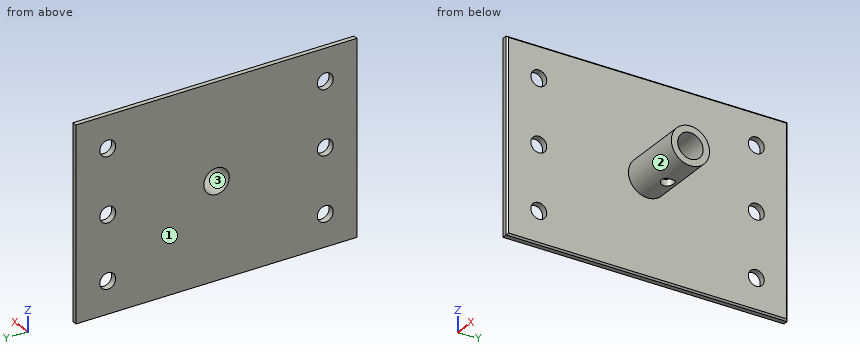
Autodesk Inventor part; units mm, degrees
ref_plane "Work Plane1" through (2, 0, -6) normal (0, 0, -1) x (-1, 0, 0)
ref_plane "YZ Plane" through (0, 0, 0) normal (1, 0, 0) x (0, 1, 0)
ref_plane "XZ Plane" through (0, 0, 0) normal (0, 1, 0) x (-1, 0, 0)
sketch "Sketch1" plane through (0, 0, 0) normal (1, 0, 0) x (0, 1, 0)
  line L0 (44.15, 30) -> (-44.15, 30)
  line L1 (-44.15, 30) -> (-44.15, -30)
  line L2 (-44.15, -30) -> (44.15, -30)
  line L3 (44.15, -30) -> (44.15, 30)
  line L4 (44.15, 30) -> (-44.15, -30) construction
  line L5 (-44.15, 30) -> (44.15, -30) construction
  circle A0 centre (0, 0) radius 4
  circle A1 centre (0, 0) radius 6
  line L6 (44.15, 30) -> (44.15, 20)
  line L7 (44.15, 20) -> (34.15, 20)
  line L8 (44.15, -30) -> (44.15, -20)
  line L9 (44.15, -20) -> (34.15, -20)
  line L10 (-44.15, 30) -> (-44.15, 20)
  line L11 (-44.15, 20) -> (-34.15, 20)
  line L12 (-44.15, -30) -> (-44.15, -20)
  line L13 (-44.15, -20) -> (-34.15, -20)
  line L14 (-44.15, 0) -> (-34.15, 0)
  line L15 (44.15, 0) -> (34.15, 0)
  circle A2 centre (34.15, 20) radius 2.5
  circle A3 centre (34.15, 0) radius 2.5
  circle A4 centre (34.15, -20) radius 2.5
  circle A5 centre (-34.15, 20) radius 2.5
  circle A6 centre (-34.15, 0) radius 2.5
  circle A7 centre (-34.15, -20) radius 2.5
  dimension "d0" = 88.3
  dimension "d1" = 60
  dimension "d2" = 8
  dimension "d3" = 12
  dimension "d4" = 10
  dimension "d5" = 10
  dimension "d6" = 10
  dimension "d7" = 10
  dimension "d8" = 10
  dimension "d9" = 10
  dimension "d10" = 10
  dimension "d11" = 10
  dimension "d12" = 10
  dimension "d13" = 10
  dimension "d14" = 5
  dimension "d15" = 5
  dimension "d16" = 5
  dimension "d17" = 5
  dimension "d18" = 5
  dimension "d19" = 5
extrude "Extrusion1" add sketch "Sketch1" along normal blind 2 contours L3 L2 L1 L0
sketch "Sketch2" plane through (2, 0, 0) normal (1, 0, 0) x (0, 0, -1)
  circle A0 centre (0, 0) radius 6
  circle A1 centre (0, 0) radius 4
  dimension "d22" = 12
  dimension "d23" = 8
extrude "Extrusion2" add sketch "Sketch2" along normal blind 21 and the other way blind 2
ref_plane "Work Plane1" through (2, 0, -6) normal (0, 0, -1) x (-1, 0, 0)
sketch "Sketch3" plane through (2, 0, -6) normal (0, 0, -1) x (-1, 0, 0)
  line L0 (-21, 6) -> (-21, -6)
  line L1 (-21, 0) -> (-10, 0)
  circle A0 centre (-10, 0) radius 2
  point P0 (2, 0)
  dimension "d28" = 11
  dimension "d29" = 4
extrude "Extrusion3" cut sketch "Sketch3" against normal blind 5
thread "Thread1"
chamfer "Chamfer1" distance 0.5 angle 45 4 edges at (2, 44.15, 0) (2, 0, -30) (2, 0, 30) (2, -44.15, 0)
properties part number "ax4_holder" material "Iron, Malleable"
Here's how the part is built. I have some questions about the finished solid (model axes, mm). Face numbers are marked on the shaded views. Coordinates: 2 decimals unless noted, no trailing zeros. Loops run counter-clockwise (first coordinate to the right, second up) from the corner with the lowest first, then second, coordinate; pieces in that order, holes last. Notation, with made-up numbers: M -23.5,75 L -0.5,75 A16 cw -0.5,104 Z; hole C 52.5,54.5 d10. An arc over 180 degrees is marked long. One line per item, written item: value.
1. Imagine slicing it at D-D (y = -9). List the corners of the cut face in (x, z) for me, and give its area (3 significant figures).
Geometry says:
outline: M 0,-30 L 1.5,-30 L 2,-29.5 L 2,29.5 L 1.5,30 L 0,30 Z
area: 120 mm2
2. Thinking about a two-plate mould opening in Y: for the marked faces 1, 2 and 3, which applies, +Y half, -Y half, draft (parallel to the pull), parting line (faces both ways), or undercut?
Geometry says:
face 1: draft
face 2: parting line
face 3: undercut
3. Will these pins go through, and if not, where does the flat tip stop? pin 1 Ø4 at (y, z) = (21, 17.5) entering from +X; pin 2 Ø1.5 at (x, z) = (3, 5) entering from -Y; pin 3 Ø4.5 at (x, y) = (12, 0) entering from -Z; pin 4 Ø6.5 at (y, z) = (34.15, 20) entering from -X.
Geometry says:
pin 1: stops at x = 2
pin 2: stops at y = -4.24
pin 3: stops at z = -6
pin 4: stops at x = 0
4. Imagine slicing it at C-C (z = 20). List the corners of the cut face in (x, y) for me, and give its area (3 significant figures).
Geometry says:
outline: M 0,-44.15 L 1.5,-44.15 L 2,-43.65 L 2,-36.65 L 0,-36.65 Z; M 0,-31.65 L 2,-31.65 L 2,31.65 L 0,31.65 Z; M 0,36.65 L 2,36.65 L 2,43.65 L 1.5,44.15 L 0,44.15 Z
area: 156 mm2
5. Imagine slicing it at A-A (y = -34.15). List the corners of the cut face in (x, z) for me.
Geometry says:
outline: M 0,-30 L 1.5,-30 L 2,-29.5 L 2,-22.5 L 0,-22.5 Z; M 0,-17.5 L 2,-17.5 L 2,-2.5 L 0,-2.5 Z; M 0,2.5 L 2,2.5 L 2,17.5 L 0,17.5 Z; M 0,22.5 L 2,22.5 L 2,29.5 L 1.5,30 L 0,30 Z
6. Imagine slicing it at B-B (z = 0). List the corners of the cut face in (x, y) for me.
Geometry says:
outline: M 0,-44.15 L 1.5,-44.15 L 2,-43.65 L 2,-36.65 L 0,-36.65 Z; M 0,-31.65 L 2,-31.65 L 2,-6 L 23,-6 L 23,-4 L 0,-4 Z; M 0,4 L 23,4 L 23,6 L 2,6 L 2,31.65 L 0,31.65 Z; M 0,36.65 L 2,36.65 L 2,43.65 L 1.5,44.15 L 0,44.15 Z
7. Please list where these lines run through material, in increasing order: probe 1 along Y at (x, z) = (9.5, 0); probe 2 along X at (y, z) = (-38.5, -4.5); probe 3 along Z at (x, y) = (14.5, 2.5).
Geometry says:
probe 1: y = -6 to -4, 4 to 6
probe 2: x = 0 to 2
probe 3: z = -5.45 to -3.12, 3.12 to 5.45
